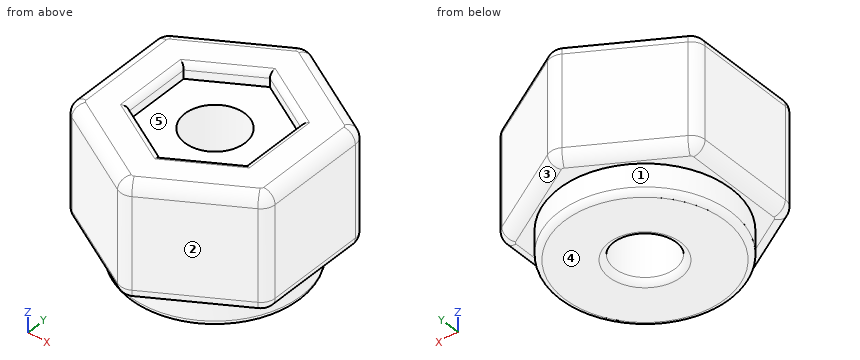
```python
from build123d import *

# Parameters (mm, degrees)
BOSS_EXTRUDE1_DEPTH = 8
CUT_EXTRUDE1_DEPTH  = 1
SKETCH3_R           = 2.1
CUT_EXTRUDE2_DEPTH  = 5
FILLET1_R           = 1
FILLET2_R           = 0.8
FILLET3_R           = 0.4
SKETCH4_R           = 6
SKETCH4_R_2         = 2.1
BOSS_EXTRUDE2_DEPTH = 2
FILLET4_R           = 0.4
SKETCH5_R           = 2.1
BOSS_EXTRUDE3_DEPTH = 0.4
SKETCH6_R           = 2.1
CUT_EXTRUDE3_DEPTH  = 14.88727504


with BuildPart() as part:
    # Sketch1 → Boss-Extrude1 (new body)
    with BuildSketch(Plane.XY):
        Polygon((0, 8.082903769), (-7, 4.041451884), (-7, -4.041451884), (0, -8.082903769), (7, -4.041451884), (7, 4.041451884), align=None)
    extrude(amount=BOSS_EXTRUDE1_DEPTH)

    # Sketch2 → Cut-Extrude1 (cut)
    with BuildSketch(Plane.XY.offset(8)):
        Polygon((0, 4.734272207), (-4.1, 2.367136104), (-4.1, -2.367136104), (0, -4.734272207), (4.1, -2.367136104), (4.1, 2.367136104), align=None)
    extrude(amount=-CUT_EXTRUDE1_DEPTH, mode=Mode.SUBTRACT)

    # Sketch3 → Cut-Extrude2 (cut)
    with BuildSketch(Plane.XY.offset(7)):
        Circle(SKETCH3_R)
    extrude(amount=-CUT_EXTRUDE2_DEPTH, mode=Mode.SUBTRACT)

    # Fillet1
    fillet1_edges = [part.edges().sort_by_distance(p)[0] for p in [
        (7, 4.041451884, 4),
        (7, -4.041451884, 4),
        (0, -8.082903769, 4),
        (-7, -4.041451884, 4),
        (-7, 4.041451884, 4),
        (0, 8.082903769, 4),
    ]]
    fillet(fillet1_edges, radius=FILLET1_R)

    # Fillet2
    fillet2_edges = [part.edges().sort_by_distance(p)[0] for p in [
        (7, 0, 0),
        (7, 0, 8),
        (3.5, 6.062177826, 0),
        (3.5, -6.062177826, 0),
        (-3.5, -6.062177826, 0),
        (-7, 0, 0),
        (-3.5, 6.062177826, 0),
        (6.866025404, 3.964101615, 0),
        (0, 7.92820323, 0),
        (-6.866025404, 3.964101615, 0),
        (-6.866025404, -3.964101615, 0),
        (0, -7.92820323, 0),
        (6.866025404, -3.964101615, 0),
        (3.5, -6.062177826, 8),
        (3.5, 6.062177826, 8),
        (-3.5, 6.062177826, 8),
        (-7, 0, 8),
        (-3.5, -6.062177826, 8),
        (6.866025404, 3.964101615, 8),
        (0, 7.92820323, 8),
        (-6.866025404, 3.964101615, 8),
        (-6.866025404, -3.964101615, 8),
        (0, -7.92820323, 8),
        (6.866025404, -3.964101615, 8),
    ]]
    fillet(fillet2_edges, radius=FILLET2_R)

    # Fillet3
    fillet3_edges = [part.edges().sort_by_distance(p)[0] for p in [
        (2.05, 3.550704156, 8),
        (-2.05, 3.550704156, 8),
        (-4.1, 0, 8),
        (-2.05, -3.550704156, 8),
        (2.05, -3.550704156, 8),
        (4.1, 0, 8),
    ]]
    fillet(fillet3_edges, radius=FILLET3_R)

    # Sketch4 → Boss-Extrude2 (add)
    with BuildSketch(Plane(origin=(0, 0, 0), x_dir=(-1, 0, 0), z_dir=(0, 0, -1))):
        with Locations(Location((0, 0, 0), (0, 0, 180))):
            Circle(SKETCH4_R)
        with Locations(Location((0, 0, 0), (0, 0, 180))):
            Circle(SKETCH4_R_2, mode=Mode.SUBTRACT)
    extrude(amount=BOSS_EXTRUDE2_DEPTH)

    # Fillet4
    fillet4_edges = [part.edges().sort_by_distance(p)[0] for p in [
        (-6, 0, -2),
        (-2.1, 0, -2),
    ]]
    fillet(fillet4_edges, radius=FILLET4_R)

    # Sketch5 → Boss-Extrude3 (add)
    with BuildSketch(Plane.XY.offset(7)):
        with Locations(Location((0, 0, 0), (0, 0, 180))):
            Circle(SKETCH5_R)
    extrude(amount=-BOSS_EXTRUDE3_DEPTH)

    # Sketch6 → Cut-Extrude3 (cut, through all)
    with BuildSketch(Plane.XY.offset(7)):
        Circle(SKETCH6_R)
    extrude(amount=-CUT_EXTRUDE3_DEPTH, mode=Mode.SUBTRACT)


solid = part.part
```
Verification items for the finished model (mm, model axes). Face numbers are marked on the shaded views. A direction names the side the tool comes from. Coordinates: 2 decimals unless noted, no trailing zeros. Write each loop counter-clockwise with the first axis right and the second up, starting at its lowest first coordinate (ties: lowest second). Pieces come first, ordered by that corner, then holes. Notation, with made-up numbers: M -39,88.25 L 2,88.25 A27 ccw 2,110.25 Z; hole C -31,67.5 d10. An arc over 180 degrees is marked long. Answer as a JSON object with one key per item and string values. Group by question number.
(1) Cross-section at A-A, the plane y = 0. Record the cut outline in (x, z), and give its area (3 significant figures).
(2) Material ranges on line 1 (X direction, y = 0, z = 4.75); line 2 (Y direction, x = 0, z = 4); line 3 (Z direction, x = -0.5, y = 2.5), recorded low to high.
(3) Release check for a two-part mould opening along X. For the marked faces 3, 4 and 5 record: +X half, -X half, draft (parallel to the pull), parting line (faces both ways), or undercut.
(4) Cross-section at B-B, the plane z = 3.75. Record the cut outline in (x, y), and give its area (3 significant figures).
(5) Tool access check on the marked faces 1 and 2. Record the directions out of +Z, -Z, +X, -X, +Y, -Y that give a thin tool (end or side, any length) a straight path to the whole face; none if there is none.
(6) Cross-section at C-C, the plane z = -1. Record the cut outline in (x, y).
(7) Gauge pin test, flat ends, axial feed: pin 1 (3 mm diameter, centred on x = -2.5, z = -0.5, fed in from +Y); pin 2 (4 mm diameter, centred on x = -3, z = 1, fed in from -Y); pin 3 (2 mm diameter, centred on x = 0, y = 3, fed in from +Z). Record the tip position at first contact, or that the pin passes through.
Reply:
{
 "1": {"outline": "M -7,0.8 A0.8 ccw -6.2,0 L -6,0 L -6,-1.6 A0.4 ccw -5.6,-2 L -2.5,-2 A0.4 ccw -2.1,-1.6 L -2.1,7 L -4.1,7 L -4.1,7.6 A0.4 ccw -4.5,8 L -6.2,8 A0.8 ccw -7,7.2 Z; M 2.1,-1.6 A0.4 ccw 2.5,-2 L 5.6,-2 A0.4 ccw 6,-1.6 L 6,0 L 6.2,0 A0.8 ccw 7,0.8 L 7,7.2 A0.8 ccw 6.2,8 L 4.5,8 A0.4 ccw 4.1,7.6 L 4.1,7 L 2.1,7 Z", "area": "89.2 mm²"},
 "2": {"line 1": "-7 to -2.1, 2.1 to 7", "line 2": "-7.93 to -2.1, 2.1 to 7.93", "line 3": "-2 to 7"},
 "3": {"face 3": "+X half", "face 4": "draft", "face 5": "undercut"},
 "4": {"outline": "M -7,-3.46 A1 ccw -6.5,-4.33 L -0.5,-7.79 A1 ccw 0.5,-7.79 L 6.5,-4.33 A1 ccw 7,-3.46 L 7,3.46 A1 ccw 6.5,4.33 L 0.5,7.79 A1 ccw -0.5,7.79 L -6.5,4.33 A1 ccw -7,3.46 Z; hole C 0,0 d4.2", "area": "156 mm²"},
 "5": {"face 1": "-Z", "face 2": "+Z, -Z, +X, -Y"},
 "6": {"outline": "C 0,0 d12; hole C 0,0 d4.2"},
 "7": {"pin 1": "y = 7.22", "pin 2": "y = -7.51", "pin 3": "z = 7"}
}
